Could you check a few things on this model? Use its own coordinates, in mm. Face numbers are marked on the shaded views. A direction names the side the tool comes from. Give positions to 0.01 mm unless a question says otherwise; leave off trailing zeros. Order: outer loops, then holes, each group sorted by start corner. A loop starts at its lowest first (then second) coordinate and runs counter-clockwise, first axis right, second up.
(1) If I drill on probe 1 along Y at (x, z) = (-0.5, 6.75); probe 2 along Z at (x, y) = (-0.75, -9.5); probe 3 along Z at (x, y) = (0, 1.05), over which ranges is the centre line in solid material (lowest first)?
(2) On a 3-axis mill with a long thin cutter (end or side, diameter ignored), from which of +Z, -Z, +X, -X, +Y, -Y can I reach the whole of each face in a straight line? I mean the marked faces 1, 2, 3 and 4. Say none if no direction works.
(3) Will these pins go through, and if not, where does the flat tip stop? pin 1 (6.5 mm diameter, centred on x = 0, z = 0, fed in from +Y); pin 2 (0.7 mm diameter, centred on x = 9, y = -3, fed in from +Z); pin 3 (6 mm diameter, centred on y = -11, z = 2.5, fed in from -X).
(4) Imagine slicing it at A-A, the plane x = 0. Write out the boundary of the cut face in (y, z), then the cut area to 3 significant figures.
(5) If we mould it in two halves opening along Y, with no side actions, what happens to the marked faces 5, 6 and 7? For each: released by +Y, released by -Y, zero draft, split by the parting line, or undercut.
(6) Imagine slicing it at B-B, the plane y = -11.5. Write out the boundary of the cut face in (x, z) (3 decimals).
(7) Imagine slicing it at C-C, the plane z = 2.5. Write out the boundary of the cut face in (x, y), then the cut area to 3 significant figures.
(8) Imagine slicing it at D-D, the plane z = 5.75. Write out the boundary of the cut face in (x, y).
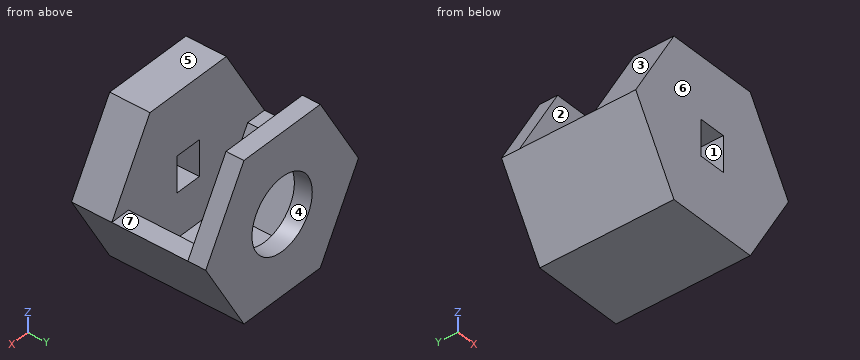
Autodesk Inventor part; units mm, degrees
ref_plane "YZ Plane" through (0, 0, 0) normal (1, 0, 0) x (0, 1, 0)
ref_plane "XZ Plane" through (0, 0, 0) normal (0, 1, 0) x (-1, 0, 0)
ref_plane "XY Plane" through (0, 0, 0) normal (0, 0, 1) x (1, 0, 0)
sketch "Sketch1" plane through (0, 0, 0) normal (0, 1, 0) x (-1, 0, 0)
  circle A0 centre (0, 0) radius 4.05
  line L0 (0, 0) -> (7.25, 0)
  line L1 (7.25, 0) -> (3.625, -6.2787)
  line L2 (3.625, -6.2787) -> (-3.625, -6.2787)
  line L3 (-3.625, -6.2787) -> (-7.25, 0)
  line L4 (-7.25, 0) -> (-3.625, 6.2787)
  line L5 (-3.625, 6.2787) -> (3.625, 6.2787)
  line L6 (3.625, 6.2787) -> (7.25, 0)
  line L7 (7.25, 0) -> (10.25, 0)
  line L8 (10.25, 0) -> (5.125, -8.8768)
  line L9 (5.125, -8.8768) -> (-5.125, -8.8768)
  line L10 (-5.125, -8.8768) -> (-10.25, 0)
  line L11 (-10.25, 0) -> (-5.125, 8.8768)
  line L12 (-5.125, 8.8768) -> (5.125, 8.8768)
  line L13 (5.125, 8.8768) -> (10.25, 0)
  line L14 (-7.25, 0) -> (-10.25, 0)
  point P0 (0, 0)
  point P1 (-10.25, 0)
  dimension "d0" = 8.1
  dimension "d1" = 7.25
  dimension "d2" = 3
extrude "Extrusion1" add sketch "Sketch1" along normal blind 2
extrude "Extrusion2" add sketch "Sketch1" against normal blind 8 contours L7 L8 L9 L10 L14 L3 L2 L1
sketch "Sketch2" plane through (0, -8, 0) normal (0, -1, 0) x (1, 0, 0)
  circle A0 centre (0, 0) radius 4.05
  line L0 (-10.25, 0) -> (-7.25, 0)
  line L1 (-7.25, 0) -> (-3.625, -6.2787)
  line L2 (-3.625, -6.2787) -> (3.625, -6.2787)
  line L3 (3.625, -6.2787) -> (7.25, 0)
  line L4 (7.25, 0) -> (10.25, 0)
  line L5 (5.125, 8.8768) -> (10.25, 0)
  line L6 (-5.125, 8.8768) -> (5.125, 8.8768)
  line L7 (-10.25, 0) -> (-5.125, 8.8768)
  line L8 (3.625, -6.2787) -> (-3.625, -6.2787)
  line L9 (-3.625, -6.2787) -> (-7.25, 0)
  line L10 (-7.25, 0) -> (-10.25, 0)
  line L11 (-10.25, 0) -> (-5.125, -8.8768)
  line L12 (-5.125, -8.8768) -> (5.125, -8.8768)
  line L13 (5.125, -8.8768) -> (10.25, 0)
  line L14 (10.25, 0) -> (7.25, 0)
  line L15 (7.25, 0) -> (3.625, -6.2787)
  line L16 (3.625, 6.2787) -> (-3.625, 6.2787)
  line L17 (-3.625, 6.2787) -> (-7.25, 0)
  line L18 (7.25, 0) -> (3.625, 6.2787)
extrude "Extrusion3" add sketch "Sketch2" along normal blind 5 contours A0 | L7 L6 L5 L4 L18 L16 L17 L0 | L0 L1 L2 L3 L4 L13 L12 L11 | L17 L16 L18 L3 L2 L1
sketch "Sketch3" plane through (0, -13, 0) normal (0, -1, 0) x (1, 0, 0)
  line L0 (0, 0) -> (1.5, 0)
  line L1 (1.5, 0) -> (-1.5, 0)
  line L2 (1.5, 0) -> (1.5, 2)
  line L3 (1.5, 2) -> (-1.5, 2)
  line L4 (-1.5, 2) -> (-1.5, -2)
  line L5 (-1.5, -2) -> (1.5, -2)
  line L6 (1.5, -2) -> (1.5, 0)
  line L7 (5.125, 8.8768) -> (-5.125, 8.8768)
  line L8 (-5.125, 8.8768) -> (-10.25, 0)
  line L9 (-10.25, 0) -> (-5.125, -8.8768)
  line L10 (-5.125, -8.8768) -> (5.125, -8.8768)
  line L11 (5.125, -8.8768) -> (10.25, 0)
  line L12 (10.25, 0) -> (5.125, 8.8768)
  dimension "d9" = 1.5
  dimension "d10" = 3
  dimension "d11" = 2
  dimension "d12" = 3
  dimension "d13" = 4
extrude "Extrusion4" cut sketch "Sketch3" against normal blind 4.5 contours L1 L4 L3 L2 L0 | L0 L6 L5 L4 L1
sketch "Sketch5" plane through (0, -8, 0) normal (0, 1, 0) x (1, 0, 0)
  circle A0 centre (0, 0) radius 4.05
  line L0 (-10.25, 0) -> (-7.25, 0)
  line L1 (-7.25, 0) -> (-3.625, 6.2787)
  line L2 (-3.625, 6.2787) -> (3.625, 6.2787)
  line L3 (3.625, 6.2787) -> (7.25, 0)
  line L4 (7.25, 0) -> (10.25, 0)
  line L5 (5.125, -8.8768) -> (10.25, 0)
  line L6 (-5.125, -8.8768) -> (5.125, -8.8768)
  line L7 (-10.25, 0) -> (-5.125, -8.8768)
  line L8 (3.625, 6.2787) -> (-3.625, 6.2787)
  line L9 (3.625, 6.2787) -> (4, 6.9282)
  line L10 (4, 6.9282) -> (8, 0)
  line L11 (8, 0) -> (4, -6.9282)
  line L12 (4, -6.9282) -> (-4, -6.9282)
  line L13 (-4, -6.9282) -> (-8, 0)
  line L14 (-8, 0) -> (-4, 6.9282)
  line L15 (-4, 6.9282) -> (4, 6.9282)
  point P0 (8, 0)
  point P1 (-8, 0)
  dimension "d19" = 0.75
extrude "Extrusion6" cut sketch "Sketch5" along normal up to surface (8 mm away) contours L14 L15 L9 L2 L1 L0 | L10 L4 L3 L9
sketch "Sketch6" plane through (0, -8, 0) normal (0, 1, 0) x (1, 0, 0)
  line L0 (-8, 0) -> (-10.25, 0)
  line L1 (-5.125, -8.8768) -> (-10.25, 0)
  line L2 (5.125, -8.8768) -> (-5.125, -8.8768)
  line L3 (10.25, 0) -> (5.125, -8.8768)
  line L4 (10.25, 0) -> (8, 0)
  line L5 (8, 0) -> (4, 6.9282)
  line L6 (4, 6.9282) -> (-4, 6.9282)
  line L7 (-4, 6.9282) -> (-8, 0)
  point P0 (0, 0)
extrude "Extrusion7" cut sketch "Sketch6" against normal up to surface (0.5 mm away)
properties part number "encoder_magnet_socket"
Answer block:
1. probe 1: y = -13 to -8.5, 0 to 2
1. probe 2: z = -8.88 to -2, 2 to 8.88
1. probe 3: z = -8.88 to -4.05, 4.05 to 8.88
2. face 1: +Y, -Y
2. face 2: +Z
2. face 3: +Z, -X, +Y, -Y
2. face 4: +Y
3. pin 1: stops at y = -8.5
3. pin 2: stops at z = 0
3. pin 3: stops at x = -10.25
4. outline: (-13, -8.88) - (2, -8.88) - (2, -4.05) - (0, -4.05) - (0, -6.93) - (-8.5, -6.93) - (-8.5, -2) - (-13, -2) - close; (-13, 2) - (-8.5, 2) - (-8.5, 8.88) - (-13, 8.88) - close; (0, 4.05) - (2, 4.05) - (2, 8.88) - (0, 8.88) - close
4. area: 97.8 mm2
5. face 5: zero draft
5. face 6: released by -Y
5. face 7: undercut
6. outline: (-10.25, 0) - (-5.125, -8.877) - (5.125, -8.877) - (10.25, 0) - (5.125, 8.877) - (-5.125, 8.877) - close; hole (-1.5, -2) - (1.5, -2) - (1.5, 2) - (-1.5, 2) - close
7. outline: (-8.81, -13) - (8.81, -13) - (8.81, -8.5) - (-8.81, -8.5) - close; (-8.81, 0) - (-3.19, 0) - (-3.19, 2) - (-8.81, 2) - close; (3.19, 0) - (8.81, 0) - (8.81, 2) - (3.19, 2) - close
7. area: 102 mm2
8. outline: (-6.93, -13) - (6.93, -13) - (6.93, -8.5) - (-6.93, -8.5) - close; (-6.93, 0) - (6.93, 0) - (6.93, 2) - (-6.93, 2) - close
